Here's how the part is built. I have some questions about the finished solid (model axes, mm). Face numbers are marked on the shaded views. A direction names the side the tool comes from. Coordinates: 2 decimals unless noted, no trailing zeros. Order: outer loops, then holes, each group sorted by start corner. A loop starts at its lowest first (then second) coordinate and runs counter-clockwise, first axis right, second up. Notation, with made-up numbers: (62.25, -39.5) -> (87.25, -39.5) arc R19 ccw to (87.25, -34.5) -> close; hole circle Ø1 at (17.25, -28). An arc over 180 degrees is marked (long way). One line per item, written item: value. Start each with the question number.
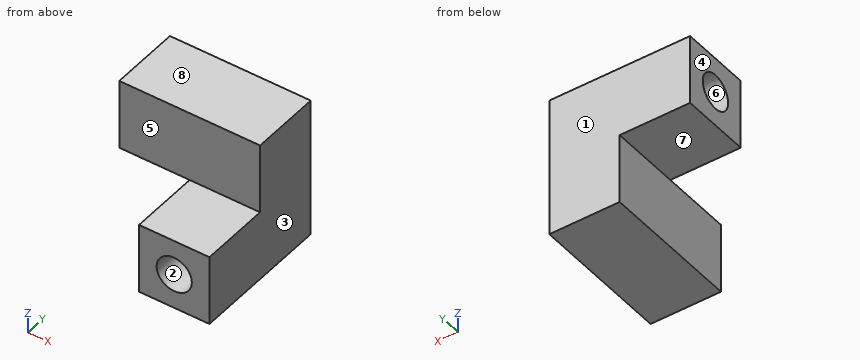
```python
from build123d import *

# Parameters (mm, degrees)
F0_W     = 25.4
F0_H     = 50.8
F1_DEPTH = 12.7
F3_W     = 25.4
F3_H     = 25.4
F3_R     = 6.35
F4_DEPTH = 50.8
F2_W     = 25.4
F2_H     = 25.4
F2_R     = 6.35
F5_DEPTH = 25.4


with BuildPart() as f1:
    # F0 (on Front) → F1 (new body, symmetric)
    with BuildSketch(Plane.XZ):
        Rectangle(F0_W, F0_H)
    extrude(amount=F1_DEPTH, both=True)

    # F3 (on face) → F4 (join)
    with BuildSketch(Plane.YZ.offset(12.7)):
        with Locations((0, 12.7)):
            Rectangle(F3_W, F3_H)
        with Locations((0, 12.7)):
            Circle(F3_R, mode=Mode.SUBTRACT)
    extrude(amount=-F4_DEPTH)

    # F2 (on face) → F5 (join)
    with BuildSketch(Plane.XZ.offset(12.7)):
        with Locations((0, -12.7)):
            Rectangle(F2_W, F2_H)
        with Locations((0, -12.7)):
            Circle(F2_R, mode=Mode.SUBTRACT)
    extrude(amount=F5_DEPTH)


solid = f1.part
```
Q1. I need wall thicknesses on line 1 (Z direction, x = 0, y = -24.25); line 2 (Z direction, x = -18.25, y = 0); line 3 (Y direction, x = -20, z = 13). Which ranges of each line are inside material? Lowest first, please.
Q2. For P1, Ø8, axis at x = -16, z = -18.5, coming from the +Y side; P2, Ø20.5, axis at x = -20, z = 9, coming from the -Y side; P3, Ø20.5, axis at x = -28, y = 4, coming from the -Z side; P4, Ø6, axis at y = 5.5, z = -5.5, coming from the -X side, each with a flat end and sliding along its axis, tell me the tip position at first contact or that it passes through.
Q3. For the marked faces 5, 6, 7 and 8, which set-ups out of +Z, -Z, +X, -X, +Y, -Y let a thin tool reach every point of the face, with its end or its side?
Q4. Imagine slicing it at D-D (x = -24). Write out the boundary of the cut face in (y, z).
Q5. Imagine slicing it at B-B (z = 12.7). Write out the boundary of the cut face in (x, y).
Q6. Imagine slicing it at A-A (y = -21.5). Write out the boundary of the cut face in (x, z).
Q7. If we mould it in two halves opening along X, with no side actions, what happens to the marked faces 1, 2, 3 and 4? For each: +X half, -X half, draft (parallel to the pull), parting line (faces both ways), or undercut.
Q8. Imagine slicing it at C-C (y = 0). Write out the boundary of the cut face in (x, z), plus the area to 3 significant figures.
Completed:
1. line 1: z = -25.4 to -19.05, -6.35 to 0
1. line 2: z = 0 to 6.35, 19.05 to 25.4
1. line 3: y = -12.7 to -6.34, 6.34 to 12.7
2. P1: stops at y = 12.7
2. P2: stops at y = -12.7
2. P3: stops at z = 0
2. P4: stops at x = -12.7
3. face 5: +Z, +X, -X, -Y
3. face 6: -X
3. face 7: -Z, -X, +Y, -Y
3. face 8: +Z, +X, -X, +Y, -Y
4. outline: (-12.7, 0) -> (12.7, 0) -> (12.7, 25.4) -> (-12.7, 25.4) -> close; hole circle Ø12.7 at (0, 12.7)
5. outline: (-38.1, -12.7) -> (12.7, -12.7) -> (12.7, 12.7) -> (-38.1, 12.7) -> (-38.1, 6.35) -> (-12.7, 6.35) -> (-12.7, -6.35) -> (-38.1, -6.35) -> close
6. outline: (-12.7, -25.4) -> (12.7, -25.4) -> (12.7, 0) -> (-12.7, 0) -> close; hole circle Ø12.7 at (0, -12.7)
7. face 1: draft
7. face 2: undercut
7. face 3: +X half
7. face 4: -X half
8. outline: (-38.1, 0) -> (-12.7, 0) -> (-12.7, -25.4) -> (12.7, -25.4) -> (12.7, 25.4) -> (-38.1, 25.4) -> (-38.1, 19.05) -> (-12.7, 19.05) -> (-12.7, 6.35) -> (-38.1, 6.35) -> close
8. area: 1,610 mm2
